Could you check a few things on this model? Use its own coordinates, in mm. Coordinates: 2 decimals unless noted, no trailing zeros. Write each loop counter-clockwise with the first axis right and the second up, starting at its lowest first coordinate (ties: lowest second). Pieces come first, ordered by that corner, then holes. Notation, with made-up numbers: M -32,46.5 L -8,46.5 A16 ccw -8,55.5 Z; hole C 7.5,30 d9. An arc over 180 degrees is marked long. Write item = value, one per line.
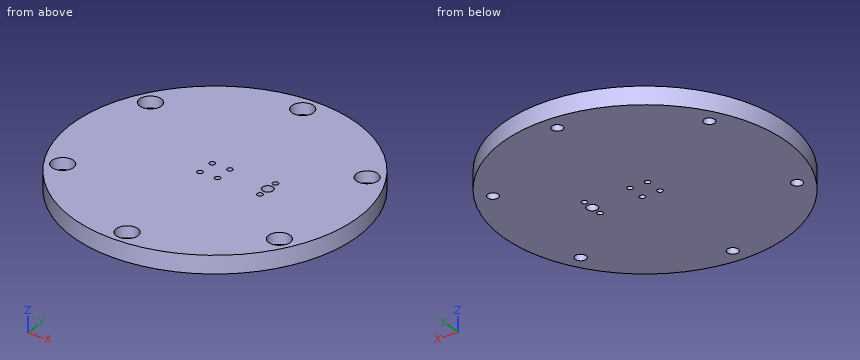
Solid Edge part; units mm, degrees
sketch "Sketch1" plane through (0, 0, 0) normal (0, 0, 1) x (1, 0, 0)
  circle A0 centre (0, 0) radius 40
extrude "Protrusion1" add sketch "Sketch1" along normal blind 5
sketch "Sketch2" plane through (0, 0, 0) normal (0, 0, 1) x (1, 0, 0)
  circle A0 centre (0, 35.5) radius 1.55
extrude "Cutout1" cut sketch "Sketch2" along normal up to next
sketch "Sketch3" plane through (0, 0, 5) normal (0, 0, 1) x (1, 0, 0)
  circle A0 centre (0, 35.5272) radius 3.05
extrude "ExtrudedCutout_2" cut sketch "Sketch3" against normal blind 3.2
pattern_circular "Pattern1" count 6 over 360 about axis through (0, 0, 5) along (0, 0, -1) of "ExtrudedCutout_2", "Cutout1"
sketch "Sketch4" plane through (0, 0, 5) normal (0, 0, 1) x (1, 0, 0)
  circle A0 centre (15, 0) radius 1.5247
extrude "ExtrudedCutout_3" cut sketch "Sketch4" against normal blind 43.3262
hole "Hole_1" at (15, -3.1469, 5) direction (0, 0, -1) diameter 1.567 end up to next thread major 2 thread length 2
hole "Hole1" at (15, 3.1469, 5) direction (0, 0, -1) diameter 1.567 end up to next thread major 2 thread length 2
hole "Hole_3" at (-2.5, -2.5, 0) direction (0, 0, 1) diameter 1.567 end up to next thread major 2 thread length 2
hole "Hole2" at (-2.5, 2.5, 0) direction (0, 0, 1) diameter 1.567 end up to next thread major 2 thread length 2
hole "Hole3" at (2.5, 2.5, 0) direction (0, 0, 1) diameter 1.567 end up to next thread major 2 thread length 2
hole "Hole4" at (2.5, -2.5, 0) direction (0, 0, 1) diameter 1.567 end up to next thread major 2 thread length 2
Item 1: Imagine slicing it at C-C (y = -17.75). Write out the boundary of the cut face in (x, z), and give its area (3 significant figures).
Numbers:
outline = M -35.85,0 L -32.29,0 L -32.29,1.8 L -33.82,1.8 L -33.82,5 L -35.85,5 Z; M -29.19,0 L 29.19,0 L 29.19,1.8 L 27.72,1.8 L 27.72,5 L -27.72,5 L -27.72,1.8 L -29.19,1.8 Z; M 32.29,0 L 35.85,0 L 35.85,5 L 33.82,5 L 33.82,1.8 L 32.29,1.8 Z
area = 308 mm²
Item 2: If I drill on line 1 along Y through (x, z) = (15, 3.6); line 2 along Y through (x, z) = (28.5, 2.2); line 3 along Y through (x, z) = (33.5, 2.1), over which ranges is the centre line in solid material (lowest first)?
Numbers:
line_1 = -37.08 to -3.93, -2.36 to -1.52, 1.52 to 2.36, 3.93 to 37.08
line_2 = -28.07 to -19.8, -15.72 to 15.72, 19.8 to 28.07
line_3 = -21.86 to -19.12, -16.41 to 16.41, 19.12 to 21.86
Item 3: Imagine slicing it at B-B (x = 0). Write out the boundary of the cut face in (y, z).
Numbers:
outline = M -40,0 L -37.05,0 L -37.05,1.8 L -38.58,1.8 L -38.58,5 L -40,5 Z; M -33.95,0 L 33.95,0 L 33.95,1.8 L 32.48,1.8 L 32.48,5 L -32.48,5 L -32.48,1.8 L -33.95,1.8 Z; M 37.05,0 L 40,0 L 40,5 L 38.58,5 L 38.58,1.8 L 37.05,1.8 Z
Item 4: Imagine slicing it at A-A (y = 0). Write out the boundary of the cut face in (x, z).
Numbers:
outline = M -40,0 L 13.48,0 L 13.48,5 L -40,5 Z; M 16.52,0 L 40,0 L 40,5 L 16.52,5 Z
Item 5: I'm going to push flat-ended pins straight in: P1, Ø2, axis at y = 16.5, z = 0.5, coming from the -X side; P2, Ø3, axis at x = -16, z = 2.5, coming from the -Y side; P3, Ø3.5, axis at x = 30.77, y = 17.76, coming from the +Z side. Where does each tip first touch, or does it pass through?
Numbers:
P1 = -36.87
P2 = -37.28
P3 = 1.8
Item 6: Imagine slicing it at D-D (z = 3.7). State how many separate pieces and enclosed holes the cut face has, and give its area (3 significant figures).
Numbers:
separate_pieces = 1
enclosed_holes = 13
area = 4,830 mm²
